Geometry check sheet. Reference: the model listing, model coordinates, mm. A direction names the side the tool comes from. Round coordinates to 2 decimals unless told otherwise and drop trailing zeros. Order: outer loops, then holes, each group sorted by start corner. A loop starts at its lowest first (then second) coordinate and runs counter-clockwise, first axis right, second up.
```python
from build123d import *

# Parameters (mm, degrees)
BOSS_EXTRUDE2_DEPTH = 10
SKETCH3_R           = 50
BOSS_EXTRUDE3_DEPTH = 10
SKETCH4_R           = 10
BOSS_EXTRUDE4_DEPTH = 90
CUT_EXTRUDE1_START  = -30
SKETCH5_R           = 10
CUT_EXTRUDE1_DEPTH  = 30
SKETCH6_R           = 13
CUT_EXTRUDE2_DEPTH  = 10
SKETCH7_R           = 10
BOSS_EXTRUDE5_DEPTH = 30
SKETCH8_R           = 20.369169003
BOSS_EXTRUDE6_DEPTH = 10
CUT_EXTRUDE3_START  = -100
SKETCH9_R           = 10
CUT_EXTRUDE3_DEPTH  = 100
SKETCH10_R          = 10
CUT_EXTRUDE4_DEPTH  = 10


with BuildPart() as part:
    # Sketch1 → Boss-Extrude2 (new body)
    with BuildSketch(Plane.XY):
        Polygon((20, 144), (-20, 144), (-20, 11.547005384), (-134.707658145, -54.679491924), (-114.707658145, -89.320508076), (0, -23.094010768), (114.707658145, -89.320508076), (134.707658145, -54.679491924), (20, 11.547005384), align=None)
    extrude(amount=BOSS_EXTRUDE2_DEPTH)

    # Sketch3 → Boss-Extrude3 (add)
    with BuildSketch(Plane.XY.offset(10)):
        with Locations((-124.707658145, -72)):
            Circle(SKETCH3_R)
        with Locations((0, 144)):
            Circle(SKETCH3_R)
        with Locations((124.707658145, -72)):
            Circle(SKETCH3_R)
    extrude(amount=-BOSS_EXTRUDE3_DEPTH)

    # Sketch4 → Boss-Extrude4 (add)
    with BuildSketch(Plane.XY.offset(10)):
        with Locations(Location((0, 144, 0), (0, 0, 180))):
            Circle(SKETCH4_R)
        with Locations(Location((124.707658145, -72, 0), (0, 0, 180))):
            Circle(SKETCH4_R)
        with Locations(Location((-124.707658145, -72, 0), (0, 0, 180))):
            Circle(SKETCH4_R)
    extrude(amount=BOSS_EXTRUDE4_DEPTH)

    # Sketch5 → Cut-Extrude1 (cut)
    with BuildSketch(Plane.XY.offset(100).offset(CUT_EXTRUDE1_START)):
        with Locations(Location((0, 144, 0), (0, 0, 180))):
            Circle(SKETCH5_R)
    extrude(amount=CUT_EXTRUDE1_DEPTH, mode=Mode.SUBTRACT)

    # Sketch6 → Cut-Extrude2 (cut)
    with BuildSketch(Plane.XY.offset(10)):
        Circle(SKETCH6_R)
    extrude(amount=-CUT_EXTRUDE2_DEPTH, mode=Mode.SUBTRACT)

    # Sketch7 → Boss-Extrude5 (add)
    with BuildSketch(Plane.XY.offset(70)):
        with Locations(Location((0, 144, 0), (0, 0, 180))):
            Circle(SKETCH7_R)
    extrude(amount=BOSS_EXTRUDE5_DEPTH)

    # Sketch8 → Boss-Extrude6 (add)
    with BuildSketch(Plane.XY.offset(10)):
        Circle(SKETCH8_R)
    extrude(amount=-BOSS_EXTRUDE6_DEPTH)

    # Sketch9 → Cut-Extrude3 (cut)
    with BuildSketch(Plane.XY.offset(100).offset(CUT_EXTRUDE3_START)):
        with Locations((-124.707658145, -72)):
            Circle(SKETCH9_R)
        with Locations((0, 144)):
            Circle(SKETCH9_R)
        with Locations((124.707658145, -72)):
            Circle(SKETCH9_R)
    extrude(amount=CUT_EXTRUDE3_DEPTH, mode=Mode.SUBTRACT)

    # Sketch10 → Cut-Extrude4 (cut)
    with BuildSketch(Plane.XY.offset(10)):
        Circle(SKETCH10_R)
    extrude(amount=-CUT_EXTRUDE4_DEPTH, mode=Mode.SUBTRACT)


solid = part.part
```
(1) Set-up check for faces 4 (the flat face through (58.036, -10.413, 4.93)), 5 (the flat face through (-14, -10, 0)), 6 (the flat face through (-20, 55, 5)): record each of +Z, -Z, +X, -X, +Y, -Y from which the full face is reachable in a straight line by a thin tool's end or side.
Returned:
face 4: +Z, -Z
face 5: -Z, +X, -X, +Y, -Y
face 6: +Z, -Z, -X
(2) Draft check along X on faces 1 (the flat face through (20, 54, 5)), 2 (the cylindrical face through (-2.17, -9.76, 5.07)), 3 (the cylindrical face through (1.911, 193.963, 5.07)). Enter one of: released by +X, released by -X, zero draft, split by the parting line, or undercut.
Returned:
face 1: released by +X
face 2: undercut
face 3: split by the parting line
(3) Sectioned sample at C-C, the plane z = 5. Record the cut outline in (x, y).
Returned:
outline: (-95.02, -31.77) arc R50 ccw (long way) to (-75.02, -66.41) - (0, -23.09) - (75.02, -66.41) arc R50 ccw (long way) to (95.02, -31.77) - (20, 11.55) - (20, 98.17) arc R50 ccw (long way) to (-20, 98.17) - (-20, 11.55) - close; hole circle Ø20 at (-124.71, -72); hole circle Ø20 at (0, 0); hole circle Ø20 at (0, 144); hole circle Ø20 at (124.71, -72)
(4) Material ranges on line 1 (X direction, y = -72, z = 7); line 2 (Y direction, x = 0, z = 4.25); line 3 (X direction, y = 140, z = 1.5), recorded low to high.
Returned:
line 1: x = -174.71 to -134.71, -114.71 to -74.71, 74.71 to 114.71, 134.71 to 174.71
line 2: y = -23.09 to -10, 10 to 134, 154 to 194
line 3: x = -49.84 to -9.17, 9.17 to 49.84
(5) Sectioned sample at B-B, the plane y = 0. Record the cut outline in (x, z).
Returned:
outline: (-40, 0) - (-10, 0) - (-10, 10) - (-40, 10) - close; (10, 0) - (40, 0) - (40, 10) - (10, 10) - close
(6) Sectioned sample at D-D, the plane x = -123. Record the cut outline in (y, z), and give its area (3 significant figures).
Returned:
outline: (-121.97, 0) - (-81.85, 0) - (-81.85, 10) - (-121.97, 10) - close; (-62.15, 0) - (-22.03, 0) - (-22.03, 10) - (-62.15, 10) - close
area: 802 mm2
(7) Sectioned sample at A-A, the plane y = -72. Record the cut outline in (x, z), and give its area (3 significant figures).
Returned:
outline: (-174.71, 0) - (-134.71, 0) - (-134.71, 10) - (-174.71, 10) - close; (-114.71, 0) - (-74.71, 0) - (-74.71, 10) - (-114.71, 10) - close; (74.71, 0) - (114.71, 0) - (114.71, 10) - (74.71, 10) - close; (134.71, 0) - (174.71, 0) - (174.71, 10) - (134.71, 10) - close
area: 1,600 mm2
(8) Depth check by flat-ended pin: P1, Ø18, axis at x = 0, y = 144, coming from the +Z side; P2, Ø5, axis at y = 56.5, z = 6.5, coming from the -X side; P3, Ø4, axis at x = 38, y = -46.5, coming from the -Z side; P4, Ø6, axis at x = 8, z = 5.5, coming from the +Y side. Enter the tip coordinate at first touch or a pass-through.
Returned:
P1: passes through
P2: stops at x = -20
P3: stops at z = 0
P4: stops at y = 193.75
